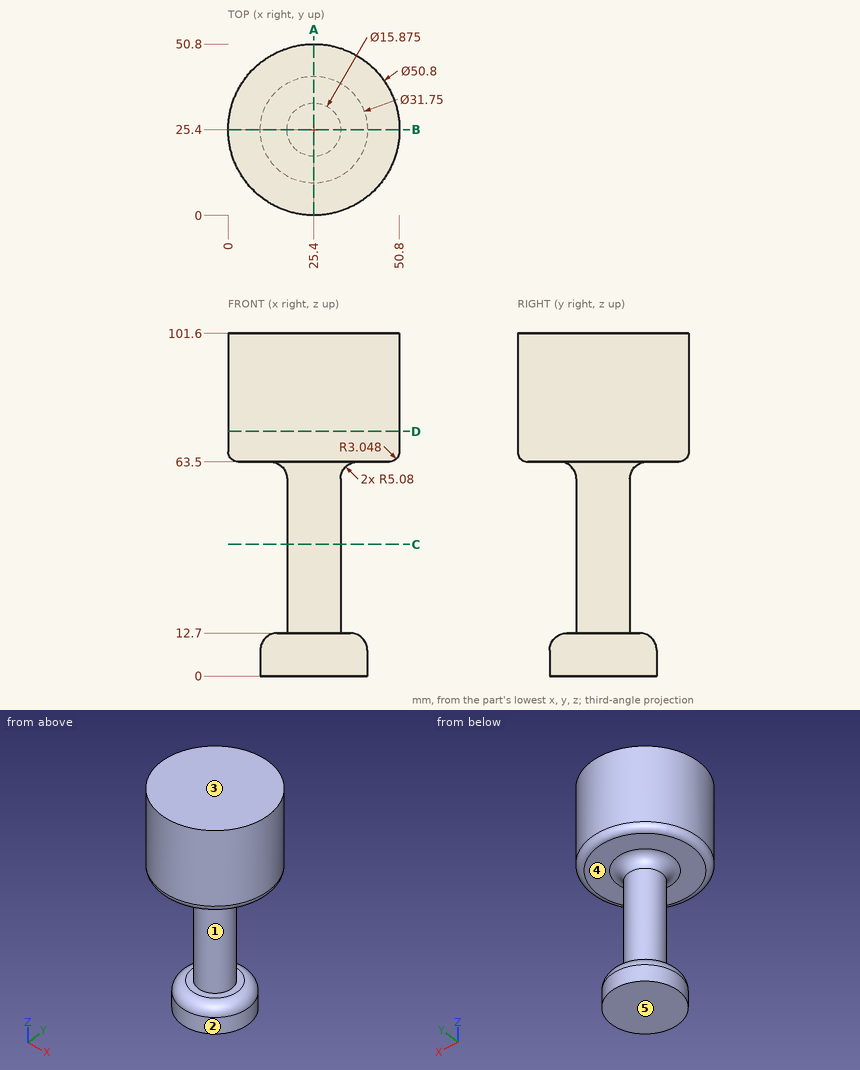
Job drawing, mm, ordinate dimensions from the low corner. One solid piece. A direction names the side the tool comes from. Give positions to 0.01 mm unless a question says otherwise; leave off trailing zeros. Loops run counter-clockwise (first coordinate to the right, second up) from the corner with the lowest first, then second, coordinate; pieces in that order, holes last. Notation, with made-up numbers: (56, -1.5) -> (111, -1.5) arc R11 ccw to (111, 12.5) -> close; hole circle Ø3 at (-34.75, 42). An arc over 180 degrees is marked (long way). Use a Markdown table: item, result. Add a question column.
(1) Wall check: line 1 along Z through (x, y) = (40, 28); line 2 along Z through (x, y) = (36.5, 25); line 3 along Z through (x, y) = (11.5, 11.5). Give the ranges that are in metal, low to high.
(2) Slice it at C-C on z = 39. List the corners of the cut face in (x, y) (1 decimal), and give its area (3 significant figures).
(3) Slice it at A-A on x = 25.4. List the corners of the cut face in (y, z) (1 decimal).
(4) Mould opens along Z. For the marked faces 1, 2 and 3 say: +Z half, -Z half, draft (parallel to the pull), parting line (faces both ways), or undercut.
(5) Tool access for the marked faces 4 and 5: list every direction of +Z, -Z, +X, -X, +Y, -Y with a clear straight run to the whole face (end or side of a thin tool).
(6) Drop flat-ended pins along their axis: pin 1 Ø6 at (x, y) = (35.5, 9.5) entering from -Z; pin 2 Ø1 at (x, z) = (35.5, 87) entering from -Y; pin 3 Ø4 at (y, z) = (39.5, 14.5) entering from +X; pin 4 Ø5 at (y, z) = (44.5, 86.5) entering from +X (3 decimals). Give the stop position or say it passes through.
(7) Slice it at D-D on z = 72.5. List the corners of the cut face in (x, y), and give its area (3 significant figures).
Filled sheet:
| question | item | result |
|---|---|---|
| 1 | line 1 | 0 to 10.71, 63.5 to 101.6 |
| 1 | line 2 | 0 to 12.69, 63.13 to 101.6 |
| 1 | line 3 | 63.5 to 101.6 |
| 2 | outline | circle Ø15.9 at (25.4, 25.4) |
| 2 | area | 198 mm2 |
| 3 | outline | (0, 66.5) arc R3 ccw to (3, 63.5) -> (12.4, 63.5) arc R5.1 cw to (17.5, 58.4) -> (17.5, 12.7) -> (14.6, 12.7) arc R5.1 ccw to (9.5, 7.6) -> (9.5, 0) -> (41.3, 0) -> (41.3, 7.6) arc R5.1 ccw to (36.2, 12.7) -> (33.3, 12.7) -> (33.3, 58.4) arc R5.1 cw to (38.4, 63.5) -> (47.8, 63.5) arc R3 ccw to (50.8, 66.5) -> (50.8, 101.6) -> (0, 101.6) -> close |
| 4 | face 1 | undercut |
| 4 | face 2 | draft |
| 4 | face 3 | +Z half |
| 5 | face 4 | none |
| 5 | face 5 | -Z, +X, -X, +Y, -Y |
| 6 | pin 1 | z = 0 |
| 6 | pin 2 | y = 1.88 |
| 6 | pin 3 | through |
| 6 | pin 4 | x = 44.625 |
| 7 | outline | circle Ø50.8 at (25.4, 25.4) |
| 7 | area | 2,030 mm2 |
